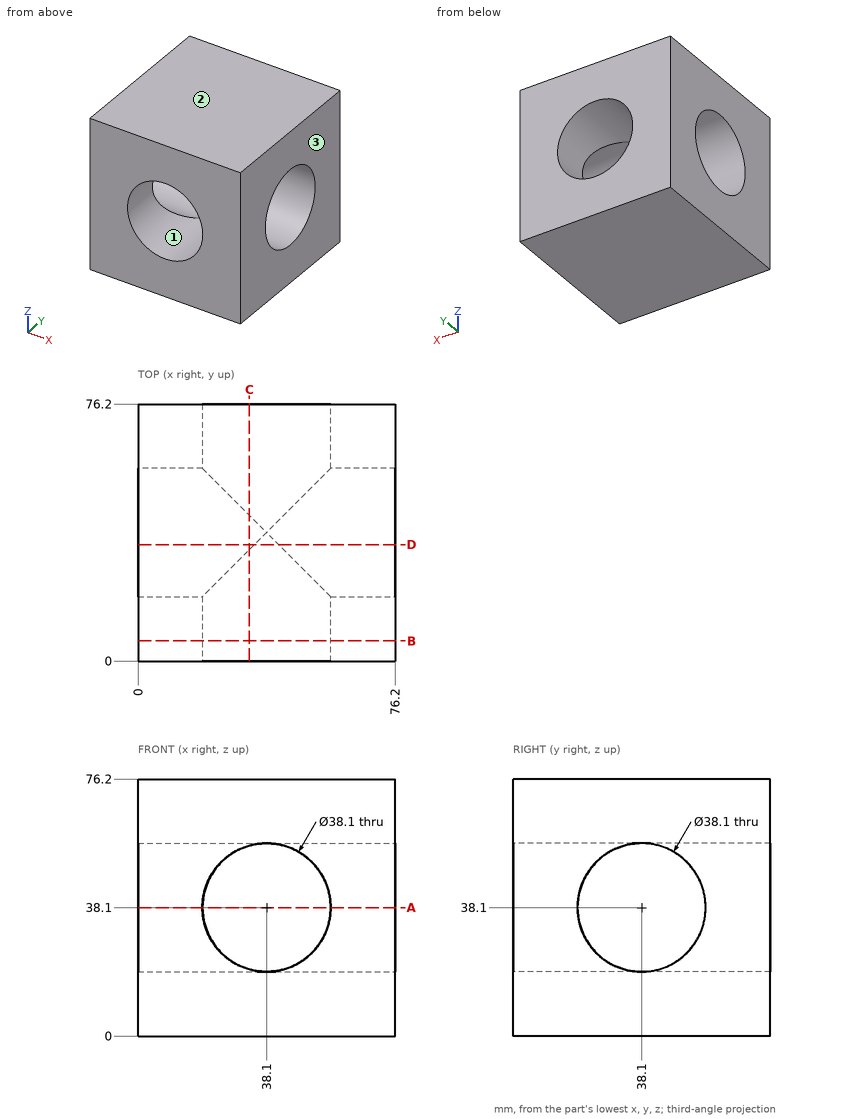
Job drawing, mm, ordinate dimensions from the low corner. One solid piece. Coordinates: 2 decimals unless noted, no trailing zeros. Order: outer loops, then holes, each group sorted by start corner. A loop starts at its lowest first (then second) coordinate and runs counter-clockwise, first axis right, second up. Notation, with made-up numbers: (23.25, 35) - (34.25, 35) arc R5 cw to (34.25, 40) - close; hole circle Ø4 at (47.25, 9). An arc over 180 degrees is marked (long way). Return JSON: item names as keys, results as strings. Group by question number.
1) Saw through at A-A, the plane z = 38.1. Write the cut outline in (x, y).
2) Saw through at C-C, the plane x = 33. Write the cut outline in (y, z).
3) Saw through at D-D, the plane y = 34.5. Write the cut outline in (x, z), plus the area to 3 significant figures.
4) Probe line 1 (Z direction, x = 29, y = 38); line 2 (Z direction, x = 41, y = 41). List the from-to ranges inside material, lowest first. Write a range as from..to.
5) Mould opens along X. For the marked faces 1, 2 and 3 say: released by +X, released by -X, zero draft, split by the parting line, or undercut.
6) Saw through at B-B, the plane y = 6. Write the cut outline in (x, z).
Values found:
{
 "1": {"outline": "(0, 0) - (19.05, 0) - (19.05, 19.05) - (0, 19.05) - close; (0, 57.15) - (19.05, 57.15) - (19.05, 76.2) - (0, 76.2) - close; (57.15, 0) - (76.2, 0) - (76.2, 19.05) - (57.15, 19.05) - close; (57.15, 57.15) - (76.2, 57.15) - (76.2, 76.2) - (57.15, 76.2) - close"},
 "2": {"outline": "(0, 0) - (76.2, 0) - (76.2, 19.75) - (43.2, 19.75) arc R19.05 cw to (33, 19.75) - (0, 19.75) - close; (0, 56.45) - (33, 56.45) arc R19.05 cw to (43.2, 56.45) - (76.2, 56.45) - (76.2, 76.2) - (0, 76.2) - close"},
 "3": {"outline": "(0, 0) - (76.2, 0) - (76.2, 19.39) - (41.7, 19.39) arc R19.05 cw to (34.5, 19.39) - (0, 19.39) - close; (0, 56.81) - (34.5, 56.81) arc R19.05 cw to (41.7, 56.81) - (76.2, 56.81) - (76.2, 76.2) - (0, 76.2) - close", "area": "2,950 mm²"},
 "4": {"line 1": "z = 0..19.05, 57.15..76.2", "line 2": "z = 0..19.27, 56.93..76.2"},
 "5": {"face 1": "undercut", "face 2": "zero draft", "face 3": "released by +X"},
 "6": {"outline": "(0, 0) - (76.2, 0) - (76.2, 76.2) - (0, 76.2) - close; hole circle Ø38.1 at (38.1, 38.1)"}
}
